from build123d import *

# Parameters (mm, degrees)
SKETCH1_R           = 4.5
BOSS_EXTRUDE1_DEPTH = 4.5
FILLET2_RADIUS      = 4.5
FILLET2_LENGTH      = 3
FILLET3_RADIUS      = 4.5
FILLET3_LENGTH      = 3
FILLET4_RADIUS      = 4.5
FILLET4_LENGTH      = 3
FILLET5_RADIUS      = 4.5
FILLET5_LENGTH      = 3
SKETCH2_R           = 2.5
CUT_EXTRUDE1_DEPTH  = 34.414068893


with BuildPart() as part:
    # Sketch1 → Boss-Extrude1 (new, symmetric)
    with BuildSketch(Plane(origin=(0, 0, 0), x_dir=(1, 0, 0), z_dir=(0, 1, 0))):
        Polygon((-26, 3), (-14, 3), (-14, -3), (-26, -3), (-26, -6), (-4.5, -6), (-4.5, -17.5), (4.5, -17.5), (4.5, -6), (26, -6), (26, -3), (14, -3), (14, 3), (26, 3), (26, 6), (4.5, 6), (4.5, 17.5), (-4.5, 17.5), (-4.5, 6), (-26, 6), align=None)
        with Locations(Location((0, 0, 0), (0, 0, 270))):
            Circle(SKETCH1_R, mode=Mode.SUBTRACT)
    extrude(amount=BOSS_EXTRUDE1_DEPTH, both=True)

    # Fillet2: full round fillet: the end face becomes a half cylinder, R = half its width
    fillet2_face = Plane((-26, 0, 4.5), x_dir=(0, 0, 1), z_dir=(-1, 0, 0))  # on the end face: x along it, z out of the body
    fillet2_slab = fillet2_face.offset(-FILLET2_RADIUS / 2) * Box(FILLET2_LENGTH, 2 * FILLET2_RADIUS, FILLET2_RADIUS, mode=Mode.PRIVATE)  # the body's end, R deep
    fillet2_round = Plane((-21.5, 0, 4.5), x_dir=(-1, 0, 0), z_dir=(0, 0, 1)) * Cylinder(FILLET2_RADIUS, FILLET2_LENGTH, mode=Mode.PRIVATE)  # its axis R under the face
    add(fillet2_slab - fillet2_round, mode=Mode.SUBTRACT)

    # Fillet3: full round fillet: the end face becomes a half cylinder, R = half its width
    fillet3_face = Plane((-26, 0, -4.5), x_dir=(0, 0, 1), z_dir=(-1, 0, 0))  # on the end face: x along it, z out of the body
    fillet3_slab = fillet3_face.offset(-FILLET3_RADIUS / 2) * Box(FILLET3_LENGTH, 2 * FILLET3_RADIUS, FILLET3_RADIUS, mode=Mode.PRIVATE)  # the body's end, R deep
    fillet3_round = Plane((-21.5, 0, -4.5), x_dir=(-1, 0, 0), z_dir=(0, 0, 1)) * Cylinder(FILLET3_RADIUS, FILLET3_LENGTH, mode=Mode.PRIVATE)  # its axis R under the face
    add(fillet3_slab - fillet3_round, mode=Mode.SUBTRACT)

    # Fillet4: full round fillet: the end face becomes a half cylinder, R = half its width
    fillet4_face = Plane((26, 0, -4.5), x_dir=(0, 0, 1), z_dir=(1, 0, 0))  # on the end face: x along it, z out of the body
    fillet4_slab = fillet4_face.offset(-FILLET4_RADIUS / 2) * Box(FILLET4_LENGTH, 2 * FILLET4_RADIUS, FILLET4_RADIUS, mode=Mode.PRIVATE)  # the body's end, R deep
    fillet4_round = Plane((21.5, 0, -4.5), x_dir=(1, 0, 0), z_dir=(0, 0, 1)) * Cylinder(FILLET4_RADIUS, FILLET4_LENGTH, mode=Mode.PRIVATE)  # its axis R under the face
    add(fillet4_slab - fillet4_round, mode=Mode.SUBTRACT)

    # Fillet5: full round fillet: the end face becomes a half cylinder, R = half its width
    fillet5_face = Plane((26, 0, 4.5), x_dir=(0, 0, -1), z_dir=(1, 0, 0))  # on the end face: x along it, z out of the body
    fillet5_slab = fillet5_face.offset(-FILLET5_RADIUS / 2) * Box(FILLET5_LENGTH, 2 * FILLET5_RADIUS, FILLET5_RADIUS, mode=Mode.PRIVATE)  # the body's end, R deep
    fillet5_round = Plane((21.5, 0, 4.5), x_dir=(1, 0, 0), z_dir=(0, 0, -1)) * Cylinder(FILLET5_RADIUS, FILLET5_LENGTH, mode=Mode.PRIVATE)  # its axis R under the face
    add(fillet5_slab - fillet5_round, mode=Mode.SUBTRACT)

    # Sketch2 → Cut-Extrude1 (cut, symmetric)
    with BuildSketch(Plane.XY.offset(-3)):
        with Locations(Location((-21.5, 0, 0), (0, 0, 180))):
            Circle(SKETCH2_R)
    cut_extrude1 = extrude(amount=CUT_EXTRUDE1_DEPTH, both=True, mode=Mode.SUBTRACT)

    # Mirror1: Cut-Extrude1 across plane
    add(cut_extrude1.mirror(Plane(origin=(0, 0, 0), x_dir=(0, 0, 1), z_dir=(1, 0, 0))), mode=Mode.SUBTRACT)


solid = part.part
Geometry: final body of the model. Coordinates: model frame, mm. A direction names the side the tool comes from. Round coordinates to 2 decimals unless told otherwise and drop trailing zeros. Write each loop counter-clockwise with the first axis right and the second up, starting at its lowest first coordinate (ties: lowest second). Pieces come first, ordered by that corner, then holes. Notation, with made-up numbers: M -4,26 L 33,26 A14 ccw 33,34 Z; hole C -2,33 d6. An arc over 180 degrees is marked long. Write item = value, one per line.
Item 1: Section query A-A on x = 20. Return loops of the section in (y, z).
Findings:
outline = M -4.5,-6 L -2,-6 L -2,-3 L -4.5,-3 Z; M -4.5,3 L -2,3 L -2,6 L -4.5,6 Z; M 2,-6 L 4.5,-6 L 4.5,-3 L 2,-3 Z; M 2,3 L 4.5,3 L 4.5,6 L 2,6 Z
Item 2: Section query B-B on y = 0. State how many separate pieces and enclosed holes the cut face has, then the cut area to 3 significant figures.
Findings:
separate_pieces = 5
enclosed_holes = 1
area = 563 mm^2
Item 3: Pin query (flat end, axial travel): P1, Ø2, axis at y = 3.5, z = -8.5, coming from the -X side; P2, Ø4, axis at x = -21.5, y = 0, coming from the -Z side; P3, Ø3, axis at x = 14.5, y = 3.5, coming from the +Z side; P4, Ø4.5, axis at y = -2, z = 14, coming from the +X side. Return the tip coordinate at first contact, or that it passes through.
Findings:
P1 = -4.5
P2 = through
P3 = 6
P4 = 4.5
Item 4: Section query D-D on x = 8.5. Return loops of the section in (y, z).
Findings:
outline = M -4.5,-6 L 4.5,-6 L 4.5,6 L -4.5,6 Z
Item 5: Access query for faces 1 (the face through (-14, 0, 0)), 2 (the face through (15, 0, 6)), 3 (the face through (4.5, 0, -12)), 4 (the face through (-4.5, 0, 12)). Directions: +Z, -Z, +X, -X, +Y, -Y. A direction counts if a zero-diameter tool reaches every point of the face in a straight line with its end or side. Return the directions, or none.
Findings:
face_1 = -X, +Y, -Y
face_2 = +Z, +X, +Y, -Y
face_3 = -Z, +X, +Y, -Y
face_4 = +Z, -X, +Y, -Y
Item 6: Material intervals for line 1 along Z through (x, y) = (23.5, 3); line 2 along Y through (x, z) = (-21.5, -3.7); line 3 along X through (y, z) = (2.5, -8.5), sorted ascending. Write a range as [from, to].
Findings:
line_1 = [-6, -3], [3, 6]
line_2 = [-4.5, -2.5], [2.5, 4.5]
line_3 = [-4.5, 4.5]
Item 7: Section query C-C on z = 0. Return loops of the section in (x, y), then the cut area to 3 significant figures.
Findings:
outline = M -14,-4.5 L -4.5,-4.5 L -4.5,4.5 L -14,4.5 Z; M 4.5,-4.5 L 14,-4.5 L 14,4.5 L 4.5,4.5 Z
area = 171 mm^2
Item 8: Pull-direction query (Y, two-part tool) for faces 5 (the face through (19, 0, -4)), 6 (the face through (0, 0, 17.5)), 7 (the face through (19, 0, 5)), 8 (the face through (-5, -4.5, 0)); classes: pulls with the +Y half, pulls with the -Y half, needs draft (parallel to the pull), parting line crosses it, or undercut.
Findings:
face_5 = undercut
face_6 = needs draft
face_7 = undercut
face_8 = pulls with the -Y half
